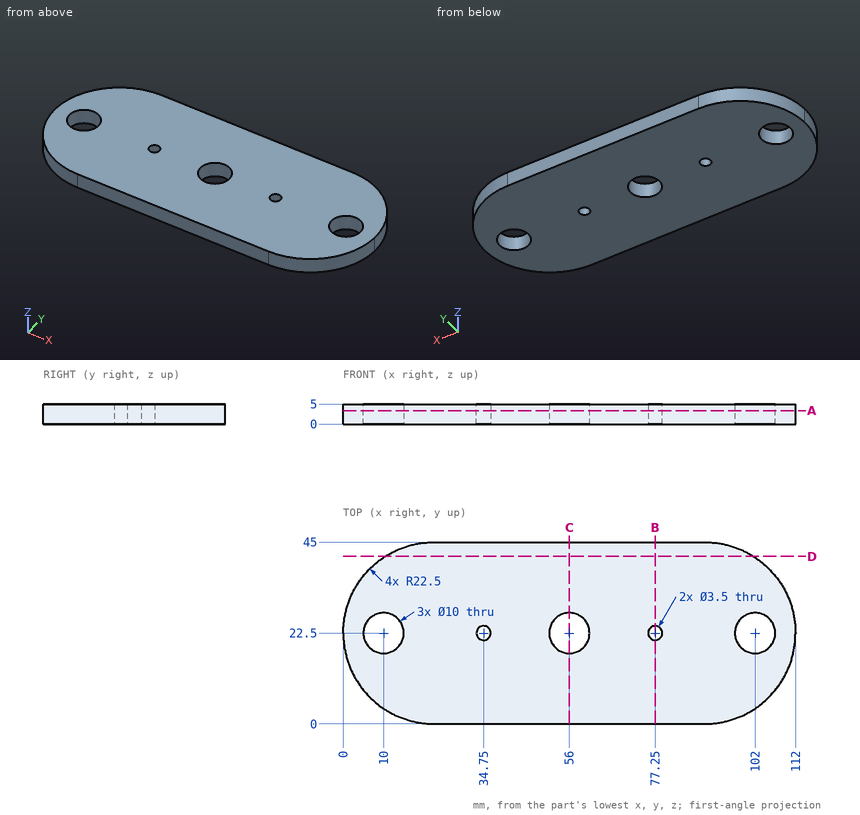
Job drawing, mm, ordinate dimensions from the low corner. One solid piece. Round coordinates to 2 decimals unless told otherwise and drop trailing zeros. Order: outer loops, then holes, each group sorted by start corner. A loop starts at its lowest first (then second) coordinate and runs counter-clockwise, first axis right, second up. Notation, with made-up numbers: M 18,-11 L 38,-11 A10 cw 38,-1 Z; hole C 47,64.5 d2. An arc over 180 degrees is marked long. Write each question's results on one line, items separated by ' | '. Start each with the question number.
(1) Saw through at B-B, the plane x = 77.25. Give the cut face in (y, z).
(2) Probe probe 1 along Y at (x, z) = (34.75, 3.8); probe 2 along Y at (x, z) = (10, 2.35); probe 3 along Y at (x, z) = (96.5, 1.3). List the from-to ranges inside material, lowest first. Write a range as from..to.
(3) Drop a flat-ended pin along its axis: pin 1 (3 mm diameter, centred on x = 34.75, y = 22.5, fed in from +Z). Give the stop position or say it passes through.
(4) Saw through at C-C, the plane x = 56. Give the cut face in (y, z).
(5) Saw through at A-A, the plane z = 3.35. State how many separate pieces and enclosed holes the cut face has, then the cut area to 3 significant figures.
(6) Saw through at D-D, the plane y = 41.5. Give the cut face in (x, z).
Established:
1) outline: M 0,0 L 20.75,0 L 20.75,5 L 0,5 Z; M 24.25,0 L 45,0 L 45,5 L 24.25,5 Z
2) probe 1: y = 0..20.75, 24.25..45 | probe 2: y = 3.79..17.5, 27.5..41.21 | probe 3: y = 1.12..43.88
3) pin 1: passes through
4) outline: M 0,0 L 17.5,0 L 17.5,5 L 0,5 Z; M 27.5,0 L 45,0 L 45,5 L 27.5,5 Z
5) separate pieces: 1 | enclosed holes: 5 | area: 4,350 mm^2
6) outline: M 10.45,0 L 101.55,0 L 101.55,5 L 10.45,5 Z
